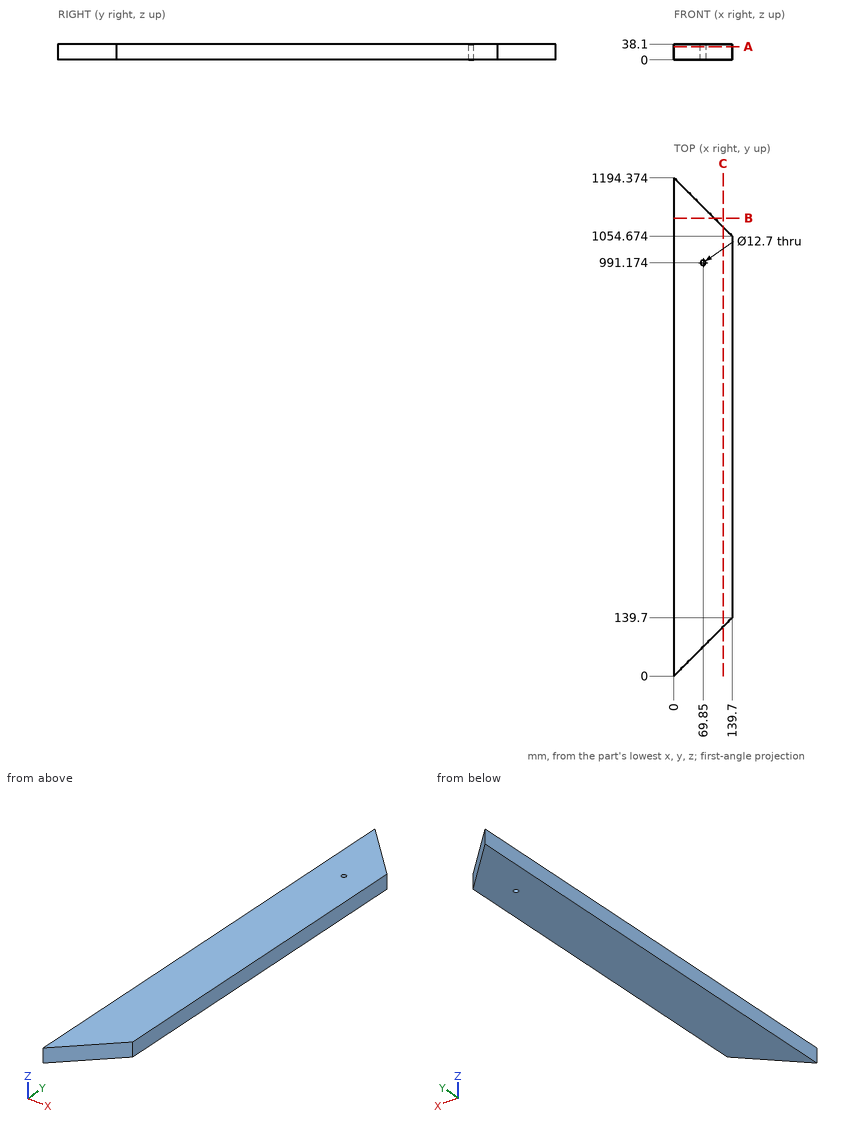
Part print with two shaded views. Sizes in mm from the minimum x, y, z corner. Give positions to 0.01 mm unless a question says otherwise; leave off trailing zeros. Write each loop counter-clockwise with the first axis right and the second up, starting at its lowest first coordinate (ties: lowest second). Pieces come first, ordered by that corner, then holes.
1) Pin check, flat tips, straight feed: pin 1 (1 mm diameter, centred on x = 112.5, z = 22.5, fed in from -Y); pin 2 (20.5 mm diameter, centred on x = 69.85, y = 991.17, fed in from -Z); pin 3 (3 mm diameter, centred on y = 127.5, z = 17, fed in from +X); pin 4 (1 mm diameter, centred on x = 96, z = 5.5, fed in from -Y). Stop position of each tip, or through.
Resolved:
pin 1: stops at y = 112
pin 2: stops at z = 0
pin 3: stops at x = 129
pin 4: stops at y = 95.5
2) Cut at C-C on x = 118. Write the cut outline in (y, z), then the cut area to 3 significant figures.
Resolved:
outline: (118, 0) - (1076.37, 0) - (1076.37, 38.1) - (118, 38.1) - close
area: 36,500 mm2
3) Cut at B-B on y = 1098. Write the cut outline in (x, z), then the cut area to 3 significant figures.
Resolved:
outline: (0, 0) - (96.37, 0) - (96.37, 38.1) - (0, 38.1) - close
area: 3,670 mm2
4) Cut at A-A on z = 31.5. Write the cut outline in (x, y).
Resolved:
outline: (0, 0) - (139.7, 139.7) - (139.7, 1054.67) - (0, 1194.37) - close; hole circle Ø12.7 at (69.85, 991.17)
5) Probe L1, parallel to Y at x = 69, z = 25; L2, parallel to Y at x = 64, z = 4.5; L3, parallel to X at y = 1071.5, z = 10.5. List the from-to ranges inside material, lowest first.
Resolved:
L1: y = 69 to 984.88, 997.47 to 1125.37
L2: y = 64 to 988.7, 993.64 to 1130.37
L3: x = 0 to 122.87
